The figure shows three views and two pictorial views of one solid part (mm, origin at its lowest corner). Answer the questions. Round coordinates to 2 decimals unless told otherwise and drop trailing zeros. Loops run counter-clockwise (first coordinate to the right, second up) from the corner with the lowest first, then second, coordinate; pieces in that order, holes last. Notation, with made-up numbers: (32.25, -31) -> (64.25, -31) arc R36 cw to (64.25, 5) -> close; hole circle Ø11 at (-21, 61). An arc over 180 degrees is marked (long way). Use a Markdown table: item, result. Add a question column.
Q1. Section A-A on z = 2.5 is taken. Give the vertices of the cut face in (x, y).
Q2. Section B-B on x = 2.75 is taken. Give the vertices of the cut face in (y, z), then the cut area to 3 significant figures.
Q3. For a pull along X with two mould halves and no side action, classify the marked faces 1, 2 and 3 as released by +X, released by -X, zero draft, split by the parting line, or undercut.
Q4. Section C-C on y = 3.25 is taken. Give the vertices of the cut face in (x, z).
Q5. Given pin 1 Ø1 at (x, y) = (2.5, 3) entering from +Z; pin 2 Ø1 at (x, y) = (9, 1.5) entering from +Z; pin 3 Ø1.5 at (x, y) = (11, 4.5) entering from +Z, each flat-ended and moving along its own axis, determine where each tip first touches the part or whether it passes through.
Q6. Section D-D on z = 5 is taken. Give the vertices of the cut face in (x, y), then the cut area to 3 significant figures.
Q7. Consider line 1 (Y direction, x = 12.75, z = 5.5); line 2 (X direction, y = 3, z = 2.5); line 3 (Z direction, x = 7.75, y = 3). Determine where each line is inside the solid, lowest interval first.
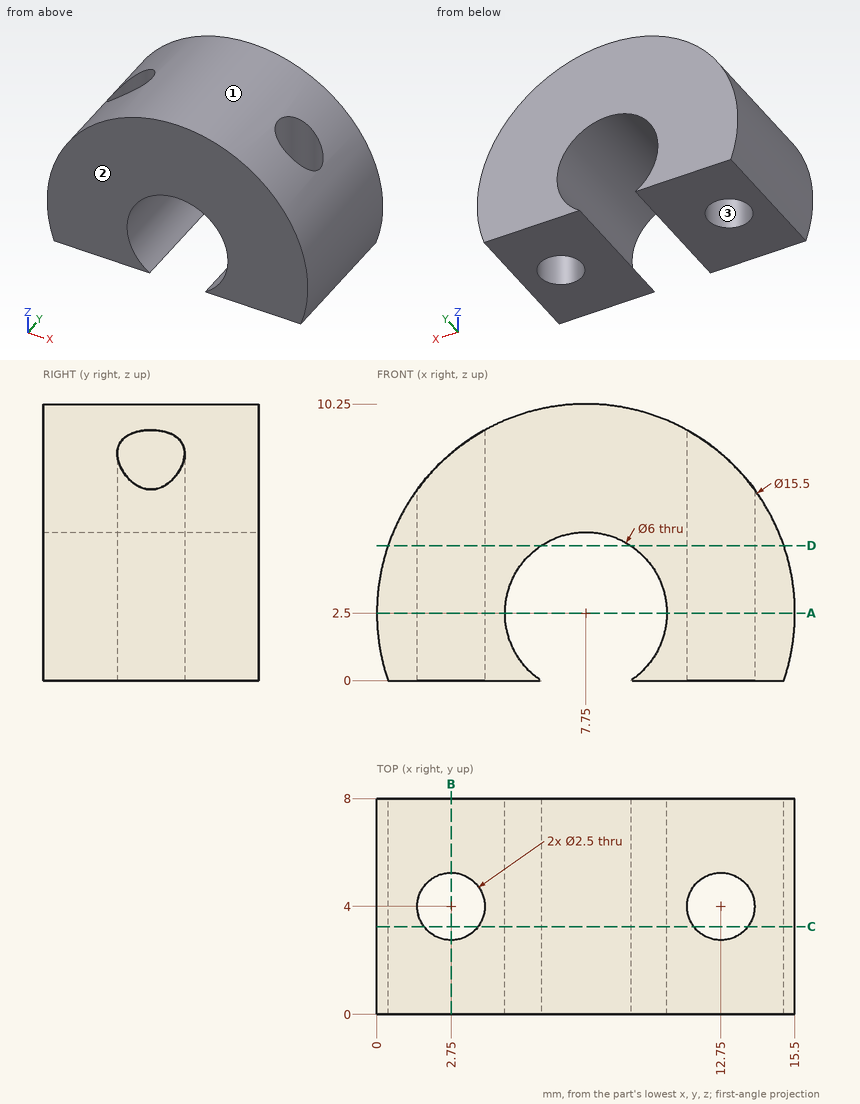
Checked values:
| question | item | result |
|---|---|---|
| 1 | outline | (0, 0) -> (4.75, 0) -> (4.75, 8) -> (0, 8) -> close; (10.75, 0) -> (15.5, 0) -> (15.5, 8) -> (10.75, 8) -> close; hole circle Ø2.5 at (2.75, 4); hole circle Ø2.5 at (12.75, 4) |
| 2 | outline | (0, 0) -> (2.75, 0) -> (2.75, 8.42) -> (0, 8.42) -> close; (5.25, 0) -> (8, 0) -> (8, 8.42) -> (5.25, 8.42) -> close |
| 2 | area | 46.3 mm2 |
| 3 | face 1 | split by the parting line |
| 3 | face 2 | zero draft |
| 3 | face 3 | undercut |
| 4 | outline | (0.41, 0) -> (1.75, 0) -> (1.75, 7.41) arc R7.75 ccw to start; (3.75, 0) -> (6.09, 0) arc R3 cw (long way) to (9.41, 0) -> (11.75, 0) -> (11.75, 9.14) arc R7.75 ccw to (3.75, 9.14) -> close; (13.75, 0) -> (15.09, 0) arc R7.75 ccw to (13.75, 7.41) -> close |
| 5 | pin 1 | stops at z = 8.58 |
| 5 | pin 2 | stops at z = 10.21 |
| 5 | pin 3 | stops at z = 9.84 |
| 6 | outline | (0.41, 0) -> (6.09, 0) -> (6.09, 8) -> (0.41, 8) -> close; (9.41, 0) -> (15.09, 0) -> (15.09, 8) -> (9.41, 8) -> close; hole circle Ø2.5 at (2.75, 4); hole circle Ø2.5 at (12.75, 4) |
| 6 | area | 81.0 mm2 |
| 7 | line 1 | y = 0 to 2.75, 5.25 to 8 |
| 7 | line 2 | x = 0 to 2, 3.5 to 4.75, 10.75 to 12, 13.5 to 15.5 |
| 7 | line 3 | z = 5.5 to 10.25 |
